from build123d import *

# Parameters (mm, degrees)
BOSS_EXTRU_1_DEPTH      = 9
ESQUISSE2_W             = 19.623971562
ESQUISSE2_H             = 15.534154535
ESQUISSE2_R             = 3
ENL_V_MAT_EXTRU_1_DEPTH = 3
ENL_V_START             = -4
ESQUISSE3_W             = 11.267201257
ESQUISSE3_H             = 13.961169169
ESQUISSE3_R             = 3
ENL_V_MAT_EXTRU_2_DEPTH = 4
CHANFREIN1_SIZE         = 4
CHANFREIN1_SIZE_2       = 2.499477408


with BuildPart() as part:
    # Esquisse1 → Boss.-Extru.1 (new body)
    with BuildSketch(Plane.XY):
        Polygon((4.041451884, 0), (2.020725942, 3.5), (-2.020725942, 3.5), (-4.041451884, 0), (-2.020725942, -3.5), (2.020725942, -3.5), align=None)
    extrude(amount=BOSS_EXTRU_1_DEPTH)

    # Esquisse2 → Enlèv. mat.-Extru.1 (cut)
    with BuildSketch(Plane.XY.offset(9)):
        with Locations((0.327116653, -1.544441398)):
            Rectangle(ESQUISSE2_W, ESQUISSE2_H)
        Circle(ESQUISSE2_R, mode=Mode.SUBTRACT)
    extrude(amount=-ENL_V_MAT_EXTRU_1_DEPTH, mode=Mode.SUBTRACT)

    # Esquisse3 → Enlèv. mat.-Extru.2 (cut)
    with BuildSketch(Plane(origin=(0, 0, 0), x_dir=(-1, 0, 0), z_dir=(0, 0, -1)).offset(ENL_V_START)):
        with Locations((0.009770186, 0.039262349)):
            Rectangle(ESQUISSE3_W, ESQUISSE3_H)
        with Locations(Location((0, 0, 0), (0, 0, 180))):
            Circle(ESQUISSE3_R, mode=Mode.SUBTRACT)
    extrude(amount=ENL_V_MAT_EXTRU_2_DEPTH, mode=Mode.SUBTRACT)

    # Chanfrein1
    # the kernel refuses this chamfer: 4, 2.499477408 mm, written as the material it takes off along each edge
    with BuildSketch(Plane(origin=(0, 0, 0), x_dir=(1, 0, 0), z_dir=(0, 1, 0))) as chanfrein1_piece_1_section:
        Polygon((3, -CHANFREIN1_SIZE), (3 - CHANFREIN1_SIZE_2, 0), (3, 0), align=None)
    chanfrein1_piece_1 = revolve(axis=Axis((0, 0, 0), (0, 0, -1)), mode=Mode.PRIVATE)
    chanfrein1_piece_1 = split(chanfrein1_piece_1, bisect_by=Plane(origin=(-1.744026904, 0, 4), z_dir=(0, 0, -1)), keep=Keep.TOP, mode=Mode.PRIVATE)
    add(chanfrein1_piece_1, mode=Mode.SUBTRACT)

    # Esquisse4 → Enlèvement de matière-Révolution1 (revolve, cut)
    with BuildSketch(Plane(origin=(0, 0, 0), x_dir=(1, 0, 0), z_dir=(0, 1, 0))):
        Polygon((0, -9), (1, -9), (1, -6.515477142), (0.2, 0), (0, 0), align=None)
    revolve(axis=Axis((0, 0, 10.381605157), (0, 0, -1)), mode=Mode.SUBTRACT)


solid = part.part
Part model, mm, in its own coordinate system. A direction names the side the tool comes from. Coordinates: 2 decimals unless noted, no trailing zeros. Loops run counter-clockwise (first coordinate to the right, second up) from the corner with the lowest first, then second, coordinate; pieces in that order, holes last. Notation, with made-up numbers: (-17.5, -7.75) -> (27.5, -7.75) arc R31 ccw to (27.5, 20.25) -> close; hole circle Ø3 at (62.5, -10). An arc over 180 degrees is marked (long way). Use a Markdown table: item, result. Add a question column.
Item 1: Which spindle directions (+Z, -Z, +X, -X, +Y, -Y) get a long thin tool onto all of the face, cutting with end or side? Do faces 1 (the cylindrical face through (-3, 0, 8)), 2 (the flat face through (3, -1.8, 5)), 3 (the flat face through (1, 3, 4)). Say none if no direction does.
Item 2: Band-saw the part on B-B on z = 7. Write the cut outline in (x, y), plus the area to 3 significant figures.
Item 3: Band-saw the part on A-A on x = 0. Write the cut outline in (y, z).
Item 4: Probe probe 1 along Y at (x, z) = (0, 7.5); probe 2 along Z at (x, y) = (2.25, 3); probe 3 along Y at (x, z) = (0.75, 8). List the from-to ranges inside material, lowest first.
Item 5: Band-saw the part on C-C on z = 1.25. Write the cut outline in (x, y), plus the area to 3 significant figures.
Item 6: Flat gauge pins, fed straight in: P1, Ø3, axis at y = -1.5, z = 1.5, coming from the +X side; P2, Ø2, axis at y = -1.5, z = 5.5, coming from the -X side; P3, Ø2, axis at x = -2.5, y = 0.5, coming from the -Z side. Where does each tip first touch, or does it go through?
Item 7: Pull direction X, two halves, no side cores. Call faces 4 (the cylindrical face through (0, 1, 8)), 5 (the conical face through (-0.255, 1.149, 1.083)), 6 (the flat face through (-1, 1, 9)), 7 (the conical face through (-0.472, 0.362, 3.212)): +X half, -X half, draft (parallel to the pull), parting line (faces both ways), or undercut.
Geometry says:
| question | item | result |
|---|---|---|
| 1 | face 1 | +Z |
| 1 | face 2 | +Z, -Z, +X, -Y |
| 1 | face 3 | -Z |
| 2 | outline | circle Ø6 at (0, 0); hole circle Ø2 at (0, 0) |
| 2 | area | 25.1 mm² |
| 3 | outline | (-3.5, 4) -> (-3, 4) -> (-0.5, 0) -> (-0.2, 0) -> (-1, 6.52) -> (-1, 9) -> (-3, 9) -> (-3, 6) -> (-3.5, 6) -> close; (0.2, 0) -> (0.5, 0) -> (3, 4) -> (3.5, 4) -> (3.5, 6) -> (3, 6) -> (3, 9) -> (1, 9) -> (1, 6.52) -> close |
| 4 | probe 1 | -3 to -1, 1 to 3 |
| 4 | probe 2 | 4 to 6 |
| 4 | probe 3 | -2.9 to -0.66, 0.66 to 2.9 |
| 5 | outline | circle Ø2.56 at (0, 0); hole circle Ø0.71 at (0, 0) |
| 5 | area | 4.77 mm² |
| 6 | P1 | x = 2.12 |
| 6 | P2 | x = -3.75 |
| 6 | P3 | z = 1.68 |
| 7 | face 4 | undercut |
| 7 | face 5 | parting line |
| 7 | face 6 | draft |
| 7 | face 7 | undercut |
